from build123d import *

# Parameters (mm, degrees)
F0_W     = 1195
F0_H     = 795
F0_R     = 130
F1_DEPTH = 15


with BuildPart() as f1:
    # F0 (on Top) → F1 (new body)
    with BuildSketch(Plane.XY):
        with Locations((444.978323, 111.086236)):
            Rectangle(F0_W, F0_H)
        with BuildLine():
            ThreePointArc((367.478323, -156.413764), (370.407255, -149.342696), (377.478323, -146.413764))
            Line((377.478323, -146.413764), (507.478323, -146.413764))
            ThreePointArc((507.478323, -146.413764), (514.549391, -149.342696), (517.478323, -156.413764))
            Line((517.478323, -156.413764), (517.478323, -196.413764))
            ThreePointArc((517.478323, -196.413764), (514.549391, -203.484832), (507.478323, -206.413764))
            Line((507.478323, -206.413764), (377.478323, -206.413764))
            ThreePointArc((377.478323, -206.413764), (370.407255, -203.484832), (367.478323, -196.413764))
            Line((367.478323, -196.413764), (367.478323, -156.413764))
        make_face(mode=Mode.SUBTRACT)
        with Locations((97.478323, -72.413764)):
            Circle(F0_R, mode=Mode.SUBTRACT)
        with Locations((444.978323, 111.086236)):
            Circle(F0_R, mode=Mode.SUBTRACT)
        with Locations((792.478323, -72.413764)):
            Circle(F0_R, mode=Mode.SUBTRACT)
        with Locations((97.478323, 294.586236)):
            Circle(F0_R, mode=Mode.SUBTRACT)
        with BuildLine():
            ThreePointArc((367.478323, 418.586236), (370.407255, 425.657304), (377.478323, 428.586236))
            Line((377.478323, 428.586236), (507.478323, 428.586236))
            ThreePointArc((507.478323, 428.586236), (514.549391, 425.657304), (517.478323, 418.586236))
            Line((517.478323, 418.586236), (517.478323, 378.586236))
            ThreePointArc((517.478323, 378.586236), (514.549391, 371.515168), (507.478323, 368.586236))
            Line((507.478323, 368.586236), (377.478323, 368.586236))
            ThreePointArc((377.478323, 368.586236), (370.407255, 371.515168), (367.478323, 378.586236))
            Line((367.478323, 378.586236), (367.478323, 418.586236))
        make_face(mode=Mode.SUBTRACT)
        with Locations((792.478323, 294.586236)):
            Circle(F0_R, mode=Mode.SUBTRACT)
    extrude(amount=F1_DEPTH)


solid = f1.part
CAD build for the part. Positions are in the model's coordinates, mm. Give positions to 0.01 mm unless a question says otherwise; leave off trailing zeros. Order: outer loops, then holes, each group sorted by start corner. A loop starts at its lowest first (then second) coordinate and runs counter-clockwise, first axis right, second up. Notation, with made-up numbers: (70, -22.75) - (80, -22.75) arc R19 cw to (80, -10.75) - close; hole circle Ø11 at (10.5, -21). An arc over 180 degrees is marked (long way). Answer in a Markdown table with one row per item.
1. Saw through at D-D, the plane x = 48.5. Give the cut face in (y, z).
Data:
| item | result |
|---|---|
| outline | (-286.41, 0) - (-192.83, 0) - (-192.83, 15) - (-286.41, 15) - close; (48.01, 0) - (174.17, 0) - (174.17, 15) - (48.01, 15) - close; (415.01, 0) - (508.59, 0) - (508.59, 15) - (415.01, 15) - close |
2. Saw through at A-A, the plane y = 182. Give the cut face in (x, z), plus the area to 3 significant figures.
Data:
| item | result |
|---|---|
| outline | (-152.52, 0) - (32.48, 0) - (32.48, 15) - (-152.52, 15) - close; (162.47, 0) - (336.02, 0) - (336.02, 15) - (162.47, 15) - close; (553.93, 0) - (727.48, 0) - (727.48, 15) - (553.93, 15) - close; (857.47, 0) - (1042.48, 0) - (1042.48, 15) - (857.47, 15) - close |
| area | 10,800 mm² |
3. Saw through at B-B, the plane x = 482.5. Give the cut face in (y, z), plus the area to 3 significant figures.
Data:
| item | result |
|---|---|
| outline | (-286.41, 0) - (-206.41, 0) - (-206.41, 15) - (-286.41, 15) - close; (-146.41, 0) - (-13.38, 0) - (-13.38, 15) - (-146.41, 15) - close; (235.55, 0) - (368.59, 0) - (368.59, 15) - (235.55, 15) - close; (428.59, 0) - (508.59, 0) - (508.59, 15) - (428.59, 15) - close |
| area | 6,390 mm² |
4. Saw through at C-C, the plane z = 10.5. Give the cut face in (x, y), plus the area to 3 significant figures.
Data:
| item | result |
|---|---|
| outline | (-152.52, -286.41) - (1042.48, -286.41) - (1042.48, 508.59) - (-152.52, 508.59) - close; hole circle Ø260 at (97.48, -72.41); hole circle Ø260 at (97.48, 294.59); hole circle Ø260 at (444.98, 111.09); hole (367.48, -196.41) arc R10 ccw to (377.48, -206.41) - (507.48, -206.41) arc R10 ccw to (517.48, -196.41) - (517.48, -156.41) arc R10 ccw to (507.48, -146.41) - (377.48, -146.41) arc R10 ccw to (367.48, -156.41) - close; hole (367.48, 378.59) arc R10 ccw to (377.48, 368.59) - (507.48, 368.59) arc R10 ccw to (517.48, 378.59) - (517.48, 418.59) arc R10 ccw to (507.48, 428.59) - (377.48, 428.59) arc R10 ccw to (367.48, 418.59) - close; hole circle Ø260 at (792.48, -72.41); hole circle Ø260 at (792.48, 294.59) |
| area | 667,000 mm² |
5. Probe probe 1 along Y at (x, z) = (446.5, 14.5); probe 2 along Y at (x, z) = (778, 9.25); probe 3 along Y at (x, z) = (194, 7.5). List the from-to ranges inside material, lowest first. Write a range as [from, to].
Data:
| item | result |
|---|---|
| probe 1 | y = [-286.41, -206.41], [-146.41, -18.9], [241.08, 368.59], [428.59, 508.59] |
| probe 2 | y = [-286.41, -201.61], [56.78, 165.39], [423.78, 508.59] |
| probe 3 | y = [-286.41, -159.5], [14.67, 207.5], [381.67, 508.59] |
6. Pull direction X, two halves, no side cores. Call faces 1 (the cylindrical face through (662.604, -66.698, 7.395)), 2 (the flat face through (304, 117, 0)): pulls with the +X half, pulls with the -X half, needs draft (parallel to the pull), parting line crosses it, or undercut.
Data:
| item | result |
|---|---|
| face 1 | undercut |
| face 2 | needs draft |
